Could you check a few things on this drawing? It's one solid part, dimensions in mm from its lowest x, y, z. Coordinates: 2 decimals unless noted, no trailing zeros. Order: outer loops, then holes, each group sorted by start corner. A loop starts at its lowest first (then second) coordinate and runs counter-clockwise, first axis right, second up. Notation, with made-up numbers: (78.5, 78.25) - (123.5, 78.25) arc R12 cw to (123.5, 91.25) - close; hole circle Ø5 at (10.5, 66). An arc over 180 degrees is marked (long way). Answer in a Markdown table with one row per item. Add a question column.
Item 1: I want a section at A-A (z = 46). Please give me the cut outline in (x, y) (3 decimals), plus the area to 3 significant figures.
Item 2: Will these pins go through, and if not, where does the flat tip stop? pin 1 Ø4 at (x, z) = (663.5, 58.5) entering from +Y; pin 2 Ø15.5 at (x, y) = (663.5, 4) entering from +Z; pin 3 Ø4 at (y, z) = (22, 97.5) entering from +X.
Item 3: I want a section at D-D (z = 109). Please give me the cut outline in (x, y).
Item 4: I want a section at C-C (z = 16). Please give me the cut outline in (x, y), plus the area to 3 significant figures.
Item 5: I want a section at B-B (y = 23). Please give me the cut outline in (x, z) (3 decimals).
Item 6: If I drill on line 1 along Z through (x, y) = (327, 4.25); line 2 along X through (y, z) = (2.75, 53.5) (3 decimals); line 3 along X through (y, z) = (25, 81) (3 decimals), over which ranges is the centre line in solid material (lowest first)? Write a range as from..to.
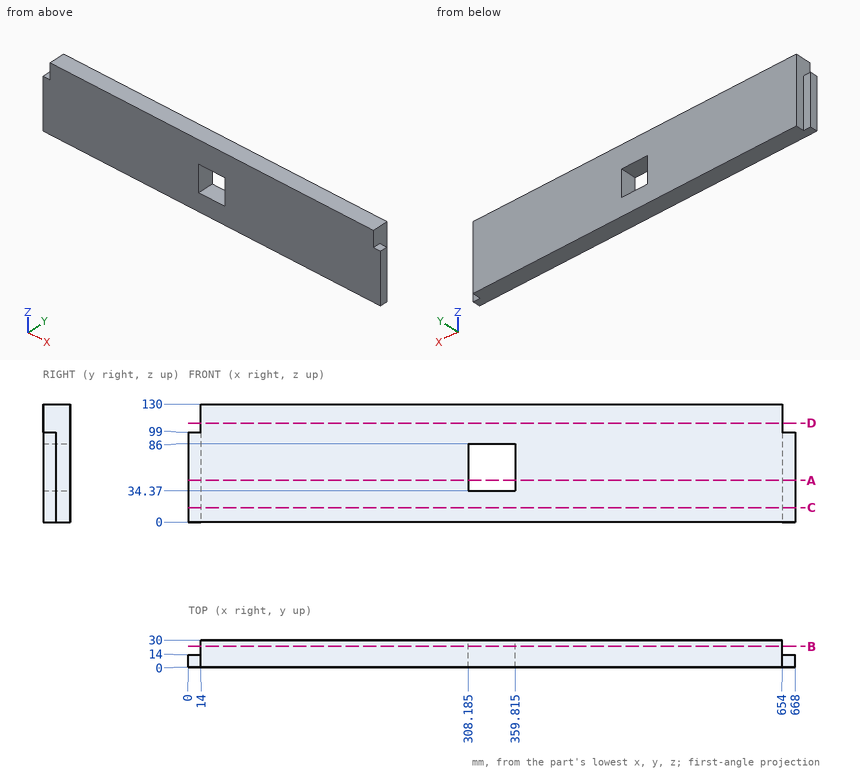
Values follow:
| question | item | result |
|---|---|---|
| 1 | outline | (0, 0) - (308.185, 0) - (308.185, 30) - (14, 30) - (14, 14) - (0, 14) - close; (359.815, 0) - (668, 0) - (668, 14) - (654, 14) - (654, 30) - (359.815, 30) - close |
| 1 | area | 18,000 mm^2 |
| 2 | pin 1 | stops at y = 14 |
| 2 | pin 2 | stops at z = 99 |
| 2 | pin 3 | stops at x = 654 |
| 3 | outline | (14, 0) - (654, 0) - (654, 30) - (14, 30) - close |
| 4 | outline | (0, 0) - (668, 0) - (668, 14) - (654, 14) - (654, 30) - (14, 30) - (14, 14) - (0, 14) - close |
| 4 | area | 19,600 mm^2 |
| 5 | outline | (14, 0) - (654, 0) - (654, 130) - (14, 130) - close; hole (308.185, 34.37) - (359.815, 34.37) - (359.815, 86) - (308.185, 86) - close |
| 6 | line 1 | z = 0..34.37, 86..130 |
| 6 | line 2 | x = 0..308.185, 359.815..668 |
| 6 | line 3 | x = 14..308.185, 359.815..654 |
